```python
from build123d import *


with BuildPart() as part:
    # Esboço1 → Revolução1 (revolve)
    with BuildSketch(Plane(origin=(0, 0, 0), x_dir=(0, 0, -1), z_dir=(1, 0, 0)), mode=Mode.PRIVATE) as revolu_o1_sk:
        Polygon((45, 25), (45, 33.94), (10, 33.94), (10, 40), (0, 40), (0, 28.575), (15.875, 28.575), (15.875, 25), align=None)
    revolve(revolu_o1_sk.sketch.rotate(Axis((0, 0, 0), (0, 0, -1)), 180), axis=Axis((0, 0, 0), (0, 0, -1)))


solid = part.part
```
CAD build for the part. Positions are in the model's coordinates, mm. A direction names the side the tool comes from. Round coordinates to 2 decimals unless told otherwise and drop trailing zeros. Write each loop counter-clockwise with the first axis right and the second up, starting at its lowest first coordinate (ties: lowest second). Pieces come first, ordered by that corner, then holes.
Item 1: Tool access for faces 5 (the cylindrical face through (-10.195, -32.373, -27.255)), 6 (the flat face through (25.3, 0.1, -15.875)), 7 (the flat face through (-27.2, 9.4, 0)): list every direction of +Z, -Z, +X, -X, +Y, -Y with a clear straight run to the whole face (end or side of a thin tool).
Filled in:
face 5: -Z
face 6: +Z
face 7: +Z, +X, -X, +Y, -Y
Item 2: Mould opens along X. For faces 1 (the cylindrical face through (-1.76, 39.96, -4.93)), 2 (the flat face through (29, -18, -10)), 3 (the cylindrical face through (-1.256, 28.547, -8.049)), 4 (the cylindrical face through (-7.509, -23.846, -30.641)) say: released by +X, released by -X, zero draft, split by the parting line, or undercut.
Filled in:
face 1: split by the parting line
face 2: zero draft
face 3: undercut
face 4: undercut
Item 3: Band-saw the part on C-C on z = -28. Write the cut outline in (x, y), then the cut area to 3 significant figures.
Filled in:
outline: circle Ø67.88 at (0, 0); hole circle Ø50 at (0, 0)
area: 1,660 mm2
Item 4: Band-saw the part on D-D on z = -8. Write the cut outline in (x, y) (3 decimals).
Filled in:
outline: circle Ø80 at (0, 0); hole circle Ø57.15 at (0, 0)
Item 5: Band-saw the part on B-B on x = 0. Write the cut outline in (y, z) (3 decimals), then the cut area to 3 significant figures.
Filled in:
outline: (-40, -10) - (-33.94, -10) - (-33.94, -45) - (-25, -45) - (-25, -15.875) - (-28.575, -15.875) - (-28.575, 0) - (-40, 0) - close; (25, -45) - (33.94, -45) - (33.94, -10) - (40, -10) - (40, 0) - (28.575, 0) - (28.575, -15.875) - (25, -15.875) - close
area: 812 mm2
Item 6: Drill centre lines: L1, parallel to X at y = 0, z = -8 (3 decimals); L2, parallel to Y at x = 1, z = -11; L3, parallel to X at y = 0, z = -38.75. Where is each one in solid material? Low to high.
Filled in:
L1: x = -40 to -28.575, 28.575 to 40
L2: y = -33.93 to -28.56, 28.56 to 33.93
L3: x = -33.94 to -25, 25 to 33.94
Item 7: Band-saw the part on A-A on y = 23.5. Write the cut outline in (x, z) (3 decimals), then the cut area to 3 significant figures.
Filled in:
outline: (-32.369, -10) - (-24.488, -10) - (-24.488, -45) - (-8.529, -45) - (-8.529, -15.875) - (-16.257, -15.875) - (-16.257, 0) - (-32.369, 0) - close; (8.529, -45) - (24.488, -45) - (24.488, -10) - (32.369, -10) - (32.369, 0) - (16.257, 0) - (16.257, -15.875) - (8.529, -15.875) - close
area: 1,350 mm2
Item 8: Drop flat-ended pins along their axis: pin 1 Ø1.5 at (y, z) = (12.5, -36.5) entering from +X; pin 2 Ø8 at (y, z) = (-6, -35) entering from +X; pin 3 Ø4 at (x, z) = (17, -4.5) entering from +Y. Give the stop position or say it passes through.
Filled in:
pin 1: stops at x = 31.84
pin 2: stops at x = 33.88
pin 3: stops at y = 37.08
